Source: CAD feature listing. Evaluate the final solid. Frame: model axes, mm. Face numbers are marked on the shaded views. A direction names the side the tool comes from. Round coordinates to 2 decimals unless told otherwise and drop trailing zeros. Loops run counter-clockwise (first coordinate to the right, second up) from the corner with the lowest first, then second, coordinate; pieces in that order, holes last. Notation, with made-up numbers: (-23, -4) - (34, -4) arc R31 ccw to (34, 24) - close; hole circle Ø3 at (8, 44). An arc over 180 degrees is marked (long way). One line per question, with ' | ' between items. Start each with the question number.
1. Ray query, line 1 (Y direction, x = -8, z = 6); line 2 (X direction, y = 0.75, z = 11); line 3 (X direction, y = -1.25, z = 8.25). Return the intervals inside material, ascending.
2. Cut plane B-B (x = -8). Return loops of the section in (y, z), then the cut area to 3 significant figures.
3. Access query for the marked faces 5 and 6. Directions: +Z, -Z, +X, -X, +Y, -Y. A direction counts if a zero-diameter tool reaches every point of the face in a straight line with its end or side. Return the directions, or none.
4. Cut plane A-A (y = 0). Return loops of the section in (x, z), then the cut area to 3 significant figures.
5. Cut plane D-D (y = 3.5). Return loops of the section in (x, z).
6. Pin query (flat end, axial travel): pin 1 (3.5 mm diameter, centred on x = 8, y = 0, fed in from -Z). Return the tip coordinate at first contact, or that it passes through.
7. Cut plane C-C (z = 11). Return loops of the section in (x, y), then the cut area to 3 significant figures.
8. Mould query, pull axis X, two halves, no side actions, for the marked faces 1, 2, 3 and 4. Classes: pulls with the +X half, pulls with the -X half, needs draft (parallel to the pull), parting line crosses it, or undercut.
```python
from build123d import *

# Parameters (mm, degrees)
SKETCH_1_W          = 46
SKETCH_1_H          = 14
EXTRUDE_1_DEPTH     = 13
CUT_EXTRUDE_1_REACH = 29.331
SKETCH_2_R          = 1.5
CUT_EXTRUDE_2_REACH = 31.9
SKETCH_3_R          = 3.65
SKETCH_4_R          = 3
CUT_EXTRUDE_3_DEPTH = 3.8


with BuildPart() as part:
    # Эскиз1 → Бобышка-Вытянуть1 (new body)
    with BuildSketch(Plane.XY):
        Rectangle(SKETCH_1_W, SKETCH_1_H)
    extrude(amount=EXTRUDE_1_DEPTH)

    # Эскиз2 → Вырез-Вытянуть1 (cut, up to next)
    with BuildSketch(Plane.XY.offset(13), mode=Mode.PRIVATE) as cut_extrude_1_sk1:
        with Locations((-8, 0)):
            Circle(SKETCH_2_R)
    cut_extrude_1_tool1 = extrude(cut_extrude_1_sk1.sketch, amount=-CUT_EXTRUDE_1_REACH, mode=Mode.PRIVATE) & part.part
    # Эскиз2 → Вырез-Вытянуть1 (cut, up to next)
    with BuildSketch(Plane.XY.offset(13), mode=Mode.PRIVATE) as cut_extrude_1_sk2:
        with Locations(Location((8, 0, 0), (0, 0, 180))):
            Circle(SKETCH_2_R)
    cut_extrude_1_tool2 = extrude(cut_extrude_1_sk2.sketch, amount=-CUT_EXTRUDE_1_REACH, mode=Mode.PRIVATE) & part.part
    add(cut_extrude_1_tool1.solids().sort_by_distance((-8, 0, 13))[0], mode=Mode.SUBTRACT)
    add(cut_extrude_1_tool2.solids().sort_by_distance((8, 0, 13))[0], mode=Mode.SUBTRACT)

    # Эскиз3 → Вырез-Вытянуть2 (cut, up to next)
    with BuildSketch(Plane(origin=(0, 7, 0), x_dir=(1, 0, 0), z_dir=(0, 1, 0)), mode=Mode.PRIVATE) as cut_extrude_2_sk1:
        with Locations((-15, -13)):
            Circle(SKETCH_3_R)
    cut_extrude_2_tool1 = extrude(cut_extrude_2_sk1.sketch, amount=-CUT_EXTRUDE_2_REACH, mode=Mode.PRIVATE) & part.part
    # Эскиз3 → Вырез-Вытянуть2 (cut, up to next)
    with BuildSketch(Plane(origin=(0, 7, 0), x_dir=(1, 0, 0), z_dir=(0, 1, 0)), mode=Mode.PRIVATE) as cut_extrude_2_sk2:
        with Locations((15, -13)):
            Circle(SKETCH_3_R)
    cut_extrude_2_tool2 = extrude(cut_extrude_2_sk2.sketch, amount=-CUT_EXTRUDE_2_REACH, mode=Mode.PRIVATE) & part.part
    add(cut_extrude_2_tool1.solids().sort_by_distance((-15, 7, 13))[0], mode=Mode.SUBTRACT)
    add(cut_extrude_2_tool2.solids().sort_by_distance((15, 7, 13))[0], mode=Mode.SUBTRACT)

    # Эскиз4 → Вырез-Вытянуть3 (cut)
    with BuildSketch(Plane(origin=(0, 0, 0), x_dir=(-1, 0, 0), z_dir=(0, 0, -1))):
        with Locations((-8, 0)):
            Circle(SKETCH_4_R)
        with Locations((8, 0)):
            Circle(SKETCH_4_R)
    extrude(amount=-CUT_EXTRUDE_3_DEPTH, mode=Mode.SUBTRACT)


solid = part.part
```
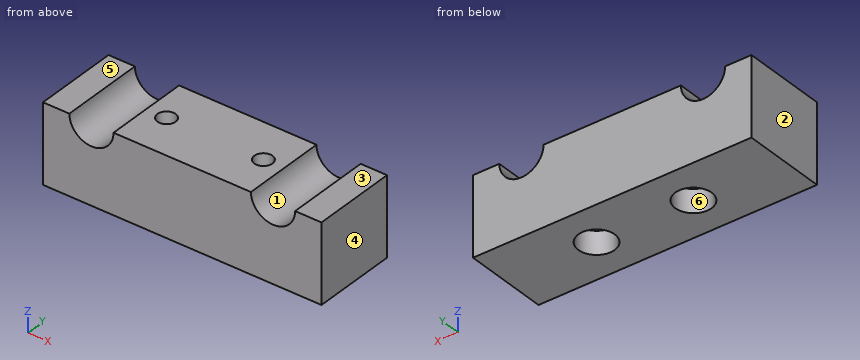
Answers follow:
1) line 1: y = -7 to -1.5, 1.5 to 7 | line 2: x = -23 to -18.05, -11.95 to -9.3, -6.7 to 6.7, 9.3 to 11.95, 18.05 to 23 | line 3: x = -23 to -8.83, -7.17 to 7.17, 8.83 to 23
2) outline: (-7, 0) - (-3, 0) - (-3, 3.8) - (-1.5, 3.8) - (-1.5, 13) - (-7, 13) - close; (1.5, 3.8) - (3, 3.8) - (3, 0) - (7, 0) - (7, 13) - (1.5, 13) - close | area: 132 mm2
3) face 5: +Z, +X, -X, +Y, -Y | face 6: -Z
4) outline: (-23, 0) - (-11, 0) - (-11, 3.8) - (-9.5, 3.8) - (-9.5, 13) - (-11.35, 13) arc R3.65 cw to (-18.65, 13) - (-23, 13) - close; (-6.5, 3.8) - (-5, 3.8) - (-5, 0) - (5, 0) - (5, 3.8) - (6.5, 3.8) - (6.5, 13) - (-6.5, 13) - close; (9.5, 3.8) - (11, 3.8) - (11, 0) - (23, 0) - (23, 13) - (18.65, 13) arc R3.65 cw to (11.35, 13) - (9.5, 13) - close | area: 455 mm2
5) outline: (-23, 0) - (23, 0) - (23, 13) - (18.65, 13) arc R3.65 cw to (11.35, 13) - (-11.35, 13) arc R3.65 cw to (-18.65, 13) - (-23, 13) - close
6) pin 1: stops at z = 3.8
7) outline: (-23, -7) - (-18.05, -7) - (-18.05, 7) - (-23, 7) - close; (-11.95, -7) - (11.95, -7) - (11.95, 7) - (-11.95, 7) - close; (18.05, -7) - (23, -7) - (23, 7) - (18.05, 7) - close; hole circle Ø3 at (-8, 0); hole circle Ø3 at (8, 0) | area: 459 mm2
8) face 1: undercut | face 2: pulls with the -X half | face 3: needs draft | face 4: pulls with the +X half
